The drawing under review shows one solid part. Ordinate dimensions are in mm from its lowest x, y, z. A direction names the side the tool comes from. Round coordinates to 2 decimals unless told otherwise and drop trailing zeros. Order: outer loops, then holes, each group sorted by start corner. A loop starts at its lowest first (then second) coordinate and runs counter-clockwise, first axis right, second up. Notation, with made-up numbers: M -5,-19 L 40,-19 A15 ccw 40,5 Z; hole C -37.75,68.25 d9. An arc over 180 degrees is marked long. Answer as a JSON object with one key per item and string values. Group by question number.
1) Consider section C-C, the plane z = 5.1. Write out the cut boundary in (x, y).
2) For the marked faces 4, 5 and 6, list the 3-axis set-ups (+Z, -Z, +X, -X, +Y, -Y) from which the entire face can be reached by the end or side of a thin tool; tool diameter is ignored.
3) The part is to be moulded in two halves that separate along Y. For the marked faces 1, 2 and 3, say which applies: +Y half, -Y half, draft (parallel to the pull), parting line (faces both ways), or undercut.
4) To check wall thickness, follow line 1 (X direction, y = 10, z = 4.1); line 2 (X direction, y = 10, z = 2.05). State the ranges of each line that lie inside material, in increasing order.
5) Insertion check: pin 1 Ø3 at (x, y) = (5.5, 5.5) entering from +Z; pin 2 Ø2.5 at (x, y) = (10, 10) entering from +Z; pin 3 Ø4 at (x, y) = (16, 5) entering from +Z. Each pin has a flat end and moves straight along its axis. Give the tip position at first contact, or say it passes through.
6) Consider section A-A, the plane x = 10. Write out the cut boundary in (y, z).
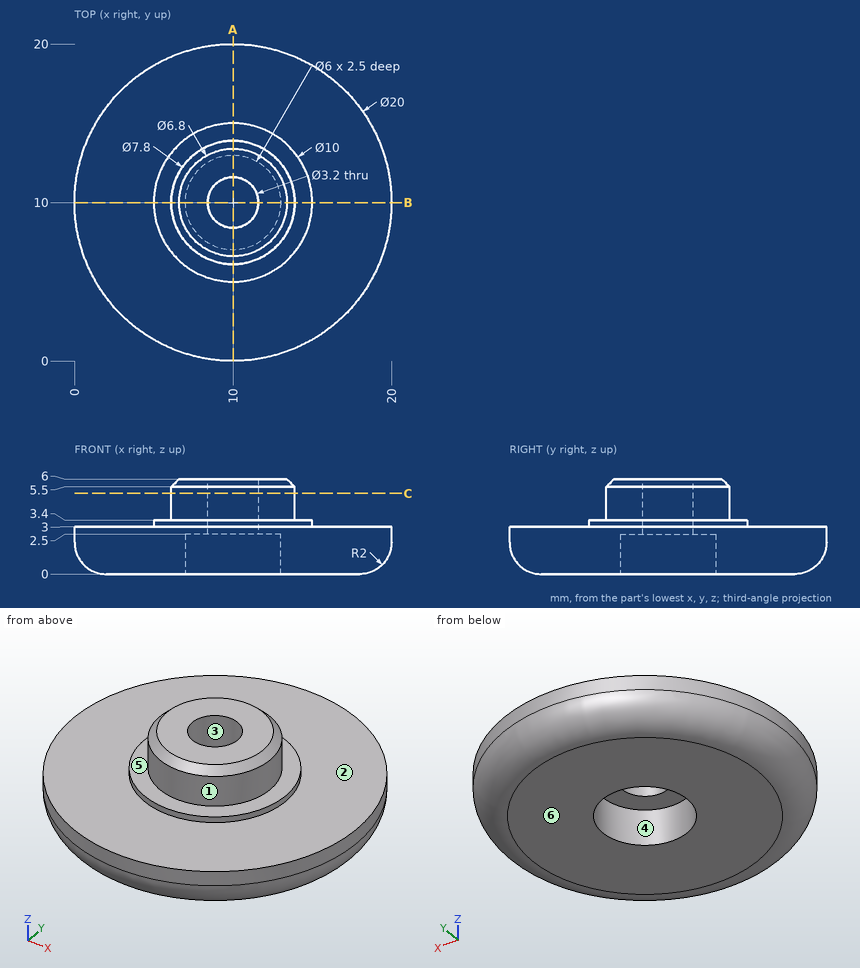
Results list:
{
 "1": {"outline": "C 10,10 d7.8; hole C 10,10 d3.2"},
 "2": {"face 4": "-Z", "face 5": "+Z", "face 6": "-Z, +X, -X, +Y, -Y"},
 "3": {"face 1": "parting line", "face 2": "draft", "face 3": "undercut"},
 "4": {"line 1": "6.1 to 8.4, 11.6 to 13.9", "line 2": "0 to 7, 13 to 20"},
 "5": {"pin 1": "z = 3.4", "pin 2": "through", "pin 3": "z = 3"},
 "6": {"outline": "M 0,2 A2 ccw 2,0 L 7,0 L 7,2.5 L 8.4,2.5 L 8.4,6 L 6.6,6 L 6.1,5.5 L 6.1,3.4 L 5,3.4 L 5,3 L 0,3 Z; M 11.6,2.5 L 13,2.5 L 13,0 L 18,0 A2 ccw 20,2 L 20,3 L 15,3 L 15,3.4 L 13.9,3.4 L 13.9,5.5 L 13.4,6 L 11.6,6 Z"}
}
